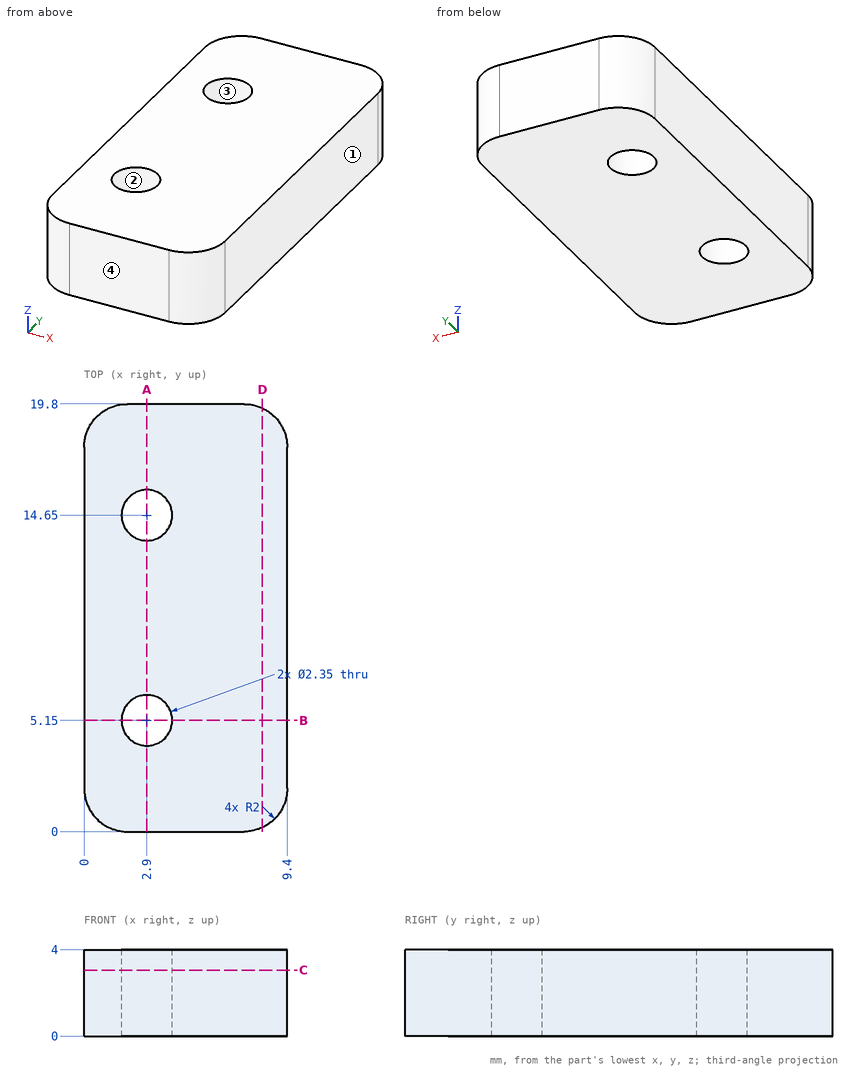
Study the drawing (mm; zero at the part's minimum x, y, z) and answer. Give positions to 0.01 mm unless a question says otherwise; leave off trailing zeros. Loops run counter-clockwise (first coordinate to the right, second up) from the corner with the lowest first, then second, coordinate; pieces in that order, holes last. Notation, with made-up numbers: (-7.5, -35.5) - (11.5, -35.5) arc R18 cw to (11.5, -2.5) - close; hole circle Ø1 at (54.5, 86.5). An arc over 180 degrees is marked (long way). Answer in a Markdown table with one row per item. Add a question column.
Q1. The part is cut by section D-D (x = 8.25). Determine the outline of the cut face in (y, z), and give its area (3 significant figures).
Q2. The part is cut by section A-A (x = 2.9). Determine the outline of the cut face in (y, z) (3 decimals).
Q3. The part is cut by section B-B (y = 5.15). Determine the outline of the cut face in (x, z) (3 decimals).
Q4. Determine the mould class of the marked faces 1, 2, 3 and 4 for opening direction Y: released by +Y, released by -Y, zero draft, split by the parting line, or undercut.
Q5. The part is cut by section C-C (z = 3.05). Determine the outline of the cut face in (x, y) (3 decimals), and give its area (3 significant figures).
Q6. Consider line 1 along Y through (x, z) = (2.9, 1.95) (3 decimals); line 2 along X through (y, z) = (5, 1.1); line 3 along X through (y, z) = (14, 0.25). Determine where each line is inside the solid, lowest interval first.
Solution:
| question | item | result |
|---|---|---|
| 1 | outline | (0.19, 0) - (19.61, 0) - (19.61, 4) - (0.19, 4) - close |
| 1 | area | 77.7 mm² |
| 2 | outline | (0, 0) - (3.975, 0) - (3.975, 4) - (0, 4) - close; (6.325, 0) - (13.475, 0) - (13.475, 4) - (6.325, 4) - close; (15.825, 0) - (19.8, 0) - (19.8, 4) - (15.825, 4) - close |
| 3 | outline | (0, 0) - (1.725, 0) - (1.725, 4) - (0, 4) - close; (4.075, 0) - (9.4, 0) - (9.4, 4) - (4.075, 4) - close |
| 4 | face 1 | zero draft |
| 4 | face 2 | undercut |
| 4 | face 3 | undercut |
| 4 | face 4 | released by -Y |
| 5 | outline | (0, 2) arc R2 ccw to (2, 0) - (7.4, 0) arc R2 ccw to (9.4, 2) - (9.4, 17.8) arc R2 ccw to (7.4, 19.8) - (2, 19.8) arc R2 ccw to (0, 17.8) - close; hole circle Ø2.35 at (2.9, 5.15); hole circle Ø2.35 at (2.9, 14.65) |
| 5 | area | 174 mm² |
| 6 | line 1 | y = 0 to 3.975, 6.325 to 13.475, 15.825 to 19.8 |
| 6 | line 2 | x = 0 to 1.73, 4.07 to 9.4 |
| 6 | line 3 | x = 0 to 1.92, 3.88 to 9.4 |
